from build123d import *

# Parameters (mm, degrees)
F0_W     = 64
F0_H     = 18
F1_DEPTH = 48
F2_W     = 32
F2_H     = 46
F3_DEPTH = 1
F5_DEPTH = 1
F7_DEPTH = 1


with BuildPart() as f1:
    # F0 (on Top) → F1 (new body)
    with BuildSketch(Plane.XY):
        with Locations((32, 9)):
            Rectangle(F0_W, F0_H)
    extrude(amount=F1_DEPTH)

    # F2 (on face) → F3 (cut)
    with BuildSketch(Plane.XZ):
        with Locations((48, 24)):
            Rectangle(F2_W, F2_H)
    extrude(amount=-F3_DEPTH, mode=Mode.SUBTRACT)

    # F4 (on face) → F5 (cut)
    with BuildSketch(Plane.XZ.offset(-1)):
        with BuildLine():
            ThreePointArc((63, 42), (61.93934, 41.56066), (61.5, 40.5))
            Line((61.5, 40.5), (61.5, 37.5))
            ThreePointArc((61.5, 37.5), (61.93934, 36.43934), (63, 36))
            Line((63, 36), (63, 42))
        make_face()
    extrude(amount=-F5_DEPTH, mode=Mode.SUBTRACT)

    # F6 (on face) → F7 (cut)
    with BuildSketch(Plane.XZ):
        with BuildLine():
            ThreePointArc((2.5, 40.5), (2.06066, 41.56066), (1, 42))
            Line((1, 42), (1, 36))
            ThreePointArc((1, 36), (2.06066, 36.43934), (2.5, 37.5))
            Line((2.5, 37.5), (2.5, 40.5))
        make_face()
    extrude(amount=-F7_DEPTH, mode=Mode.SUBTRACT)


solid = f1.part
Geometry: final body of the model. Coordinates: model frame, mm. A direction names the side the tool comes from. Round coordinates to 2 decimals unless told otherwise and drop trailing zeros. Loops run counter-clockwise (first coordinate to the right, second up) from the corner with the lowest first, then second, coordinate; pieces in that order, holes last. Notation, with made-up numbers: M -24,66.25 L -3,66.25 A15 cw -3,85.25 Z; hole C 42.5,2.25 d5. An arc over 180 degrees is marked long. Put each result on its own line as item: value. Start each with the question number.
(1) Draft query along Z for faces 4 (the face through (32, 9, 48)), 5 (the face through (32, 18, 24)), 6 (the face through (62, 2, 39)). Return one class per face: +Z half, -Z half, draft (parallel to the pull), parting line (faces both ways), or undercut.
(2) Contact query for flat-ended pins moving along their axis: pin 1 Ø5 at (x, z) = (53.5, 15) entering from -Y; pin 2 Ø0.5 at (y, z) = (0.5, 40) entering from +X; pin 3 Ø0.8 at (x, z) = (62, 38.5) entering from -Y. Output: stop coordinate, or through.
(3) Material intervals for line 1 along Y through (x, z) = (59.5, 26), sorted ascending. Write a range as [from, to].
(4) Section query B-B (z = 7). Return loops of the section in (x, y), then the cut area to 3 significant figures.
(5) Set-up query: faces 1 (the face through (2, 1, 39)), 2 (the face through (48, 1, 24)), 3 (the face through (64, 11, 24)). Return all of +Z, -Z, +X, -X, +Y, -Y with unobstructed straight access to the full face (end or side cutting, diameter ignored); none if empty.
(6) Section query A-A (x = 41). Return loops of the section in (y, z).
Findings below:
1. face 4: +Z half
1. face 5: draft
1. face 6: undercut
2. pin 1: stops at y = 1
2. pin 2: stops at x = 32
2. pin 3: stops at y = 2
3. line 1: y = [1, 18]
4. outline: M 0,0 L 32,0 L 32,1 L 64,1 L 64,18 L 0,18 Z
4. area: 1,120 mm2
5. face 1: -Y
5. face 2: +X, -Y
5. face 3: +Z, -Z, +X, +Y, -Y
6. outline: M 0,0 L 18,0 L 18,48 L 0,48 L 0,47 L 1,47 L 1,1 L 0,1 Z
